Here's how the part is built. I have some questions about the finished solid (model axes, mm). Give positions to 0.01 mm unless a question says otherwise; leave off trailing zeros. Loops run counter-clockwise (first coordinate to the right, second up) from the corner with the lowest first, then second, coordinate; pieces in that order, holes last. Notation, with made-up numbers: (-39, 6) - (-32, 6) arc R14 cw to (-32, 22) - close; hole circle Ø6 at (51.5, 17). An arc over 180 degrees is marked (long way). Return JSON: item names as keys, results as strings. Group by question number.
(1) If we section it at A-A (z = 2.95): Please give me the cut outline in (x, y).
(2) If we section it at D-D (z = 0.9): Please give me the cut outline in (x, y), then the cut area to 3 significant figures.
(3) If we section it at B-B (x = 5.3): Please give me the cut outline in (y, z), then the cut area to 3 significant figures.
(4) I need wall thicknesses on probe 1 along X at (y, z) = (-0.7, 2.95); probe 2 along X at (y, z) = (-1, 2.95); probe 3 along Y at (x, z) = (9.75, 4.8). Which ranges of each line are inside material? Lowest first, please. Write a range as [from, to].
(5) If we section it at C-C (y = -2.45): Please give me the cut outline in (x, z).
(6) For P1, Ø1.5, axis at y = -1, z = 5, coming from the -X side, with a flat end and sliding along its axis, tell me the tip position at first contact or that it passes through.
```python
from build123d import *

# Parameters (mm, degrees)
EXTRUDE_1_DEPTH     = 5.9
SKETCH_2_R          = 1.3
CUT_EXTRUDE_1_DEPTH = 5.9


with BuildPart() as part:
    # 草图1 → 凸台-拉伸1 (new body)
    with BuildSketch(Plane.XY):
        Polygon((0, 0), (10.6, 0), (8.45, -2.8), (2.15, -2.8), align=None)
    extrude(amount=EXTRUDE_1_DEPTH)

    # 草图2 → 切除-拉伸1 (cut)
    with BuildSketch(Plane(origin=(0, 0, 0), x_dir=(1, 0, 0), z_dir=(0, 1, 0))):
        with Locations(Location((5.3, -2.95, 0), (0, 0, 270))):
            Circle(SKETCH_2_R)
    extrude(amount=-CUT_EXTRUDE_1_DEPTH, mode=Mode.SUBTRACT)


solid = part.part
```
Values:
{
 "1": {"outline": "(0, 0) - (2.15, -2.8) - (4, -2.8) - (4, 0) - close; (6.6, -2.8) - (8.45, -2.8) - (10.6, 0) - (6.6, 0) - close"},
 "2": {"outline": "(0, 0) - (2.15, -2.8) - (8.45, -2.8) - (10.6, 0) - close", "area": "23.7 mm2"},
 "3": {"outline": "(-2.8, 0) - (0, 0) - (0, 1.65) - (-2.8, 1.65) - close; (-2.8, 4.25) - (0, 4.25) - (0, 5.9) - (-2.8, 5.9) - close", "area": "9.24 mm2"},
 "4": {"probe 1": "[0.54, 4], [6.6, 10.06]", "probe 2": "[0.77, 4], [6.6, 9.83]", "probe 3": "[-1.11, 0]"},
 "5": {"outline": "(1.88, 0) - (8.72, 0) - (8.72, 5.9) - (1.88, 5.9) - close; hole circle Ø2.6 at (5.3, 2.95)"},
 "6": {"P1": "x = 0.19"}
}
